```python
from build123d import *

# Parameters (mm, degrees)
F0_R     = 20
F1_DEPTH = 10
F3_R     = 2.5
F4_DEPTH = 5
F6_COUNT = 12


with BuildPart() as f1:
    # F0 (on Top) → F1 (new body)
    with BuildSketch(Plane.XY):
        Circle(F0_R)
    extrude(amount=F1_DEPTH)


with BuildPart() as f4:
    # F3 (on offset) → F4 (new body)
    with BuildSketch(Plane.XZ.offset(20)):
        with Locations((0, 5)):
            Circle(F3_R)
    extrude(amount=-F4_DEPTH)


with BuildPart() as f6_1:
    # F6: instance of F4
    add(f4.part.rotate(Axis((0, 0, 0), (0, 0, -1)), 1 * 360 / F6_COUNT))


with BuildPart() as f6_2:
    # F6: instance of F4
    add(f4.part.rotate(Axis((0, 0, 0), (0, 0, -1)), 2 * 360 / F6_COUNT))


with BuildPart() as f6_3:
    # F6: instance of F4
    add(f4.part.rotate(Axis((0, 0, 0), (0, 0, -1)), 3 * 360 / F6_COUNT))


with BuildPart() as f6_4:
    # F6: instance of F4
    add(f4.part.rotate(Axis((0, 0, 0), (0, 0, -1)), 4 * 360 / F6_COUNT))


with BuildPart() as f6_5:
    # F6: instance of F4
    add(f4.part.rotate(Axis((0, 0, 0), (0, 0, -1)), 5 * 360 / F6_COUNT))


with BuildPart() as f6_6:
    # F6: instance of F4
    add(f4.part.rotate(Axis((0, 0, 0), (0, 0, -1)), 6 * 360 / F6_COUNT))


with BuildPart() as f6_7:
    # F6: instance of F4
    add(f4.part.rotate(Axis((0, 0, 0), (0, 0, -1)), 7 * 360 / F6_COUNT))


with BuildPart() as f6_8:
    # F6: instance of F4
    add(f4.part.rotate(Axis((0, 0, 0), (0, 0, -1)), 8 * 360 / F6_COUNT))


with BuildPart() as f6_9:
    # F6: instance of F4
    add(f4.part.rotate(Axis((0, 0, 0), (0, 0, -1)), 9 * 360 / F6_COUNT))


with BuildPart() as f6_10:
    # F6: instance of F4
    add(f4.part.rotate(Axis((0, 0, 0), (0, 0, -1)), 10 * 360 / F6_COUNT))


with BuildPart() as f6_11:
    # F6: instance of F4
    add(f4.part.rotate(Axis((0, 0, 0), (0, 0, -1)), 11 * 360 / F6_COUNT))


with BuildPart() as f1_1:
    add(f1.part)

    # F7: cut F6_2, F6_1, F4, F6_11, F6_3, F6_9, F6_10, F6_8, F6_4, F6_5, F6_6, F6_7
    add(f6_2.part, mode=Mode.SUBTRACT)
    add(f6_1.part, mode=Mode.SUBTRACT)
    add(f4.part, mode=Mode.SUBTRACT)
    add(f6_11.part, mode=Mode.SUBTRACT)
    add(f6_3.part, mode=Mode.SUBTRACT)
    add(f6_9.part, mode=Mode.SUBTRACT)
    add(f6_10.part, mode=Mode.SUBTRACT)
    add(f6_8.part, mode=Mode.SUBTRACT)
    add(f6_4.part, mode=Mode.SUBTRACT)
    add(f6_5.part, mode=Mode.SUBTRACT)
    add(f6_6.part, mode=Mode.SUBTRACT)
    add(f6_7.part, mode=Mode.SUBTRACT)


solid = f1_1.part
```
Geometry: final body of the model. Coordinates: model frame, mm. A direction names the side the tool comes from. Round coordinates to 2 decimals unless told otherwise and drop trailing zeros. Loops run counter-clockwise (first coordinate to the right, second up) from the corner with the lowest first, then second, coordinate; pieces in that order, holes last. Notation, with made-up numbers: (77.25, 55) -> (111.25, 55) arc R21 cw to (111.25, 87) -> close; hole circle Ø7 at (-32, 71). An arc over 180 degrees is marked (long way). Write each question's results on one line, items separated by ' | '.
Item 1: Set-up query: faces 1 (the face through (12.973, -7.53, 5.035)), 2 (the face through (-0.33, -17.54, 7.48)), 3 (the face through (0.33, 17.54, 7.48)). Return all of +Z, -Z, +X, -X, +Y, -Y with unobstructed straight access to the full face (end or side cutting, diameter ignored); none if empty.
Answers below:
face 1: none | face 2: -Y | face 3: +Y
Item 2: Line query: probe 1 along Y at (x, z) = (-13, 2.75); probe 2 along X at (y, z) = (-14.5, 3); probe 3 along Z at (x, y) = (0, 16). Output: solid intervals per line, ascending. Write a range as [from, to].
Answers below:
probe 1: y = [-15.2, -8.76], [-7.48, 7.48], [8.76, 15.2] | probe 2: x = [-13.77, -10.1], [-6.64, 6.64], [10.1, 13.77] | probe 3: z = [0, 2.5], [7.5, 10]
Item 3: Cut plane D-D on x = -6.5. State how many separate pieces and enclosed holes the cut face has, and give its area (3 significant figures).
Answers below:
separate pieces: 1 | enclosed holes: 2 | area: 361 mm²
Item 4: Pin query (flat end, axial travel): pin 1 Ø4 at (x, z) = (7, 6) entering from -Y; pin 2 Ø3 at (x, z) = (-1.5, 4.5) entering from -Y; pin 3 Ø4 at (y, z) = (0, 5) entering from -X. Return the tip coordinate at first contact, or that it passes through.
Answers below:
pin 1: stops at y = -19.36 | pin 2: stops at y = -19.94 | pin 3: stops at x = -15
Item 5: Cut plane C-C on z = 1. Return the cut outline in (x, y), and give its area (3 significant figures).
Answers below:
outline: circle Ø40 at (0, 0) | area: 1,260 mm²
Item 6: Cut plane A-A on x = 0. Return the cut outline in (y, z), and give its area (3 significant figures).
Answers below:
outline: (-20, 0) -> (20, 0) -> (20, 2.5) -> (15, 2.5) -> (15, 7.5) -> (20, 7.5) -> (20, 10) -> (-20, 10) -> (-20, 7.5) -> (-15, 7.5) -> (-15, 2.5) -> (-20, 2.5) -> close | area: 350 mm²
Item 7: Pull-direction query (Y, two-part tool) for faces 4 (the face through (15, 0, 5)), 5 (the face through (14.26, -10.36, 6.69)), 6 (the face through (0, 0, 0)), 7 (the face through (-4.336, -19.524, 4.93)); classes: pulls with the +Y half, pulls with the -Y half, needs draft (parallel to the pull), parting line crosses it, or undercut.
Answers below:
face 4: undercut | face 5: undercut | face 6: needs draft | face 7: parting line crosses it
